from build123d import *

# Parameters (mm, degrees)
SKIZZE1_W                            = 57
SKIZZE1_H                            = 123
AUFSATZ_LINEAR_AUSTRAGEN1_DEPTH      = 2.5
SCHNITT_LINEAR_AUSTRAGEN1_DEPTH      = 84.889808678
SCHNITT_LINEAR_AUSTRAGEN2_DEPTH      = 68.828828679
SCHNITT_LINEAR_AUSTRAGEN3_DEPTH      = 70.726045338
SCHNITT_LINEAR_AUSTRAGEN3_DEPTH_BACK = 70.726045338
SCHNITT_LINEAR_AUSTRAGEN4_DEPTH      = 70.47454308
SCHNITT_LINEAR_AUSTRAGEN4_DEPTH_BACK = 70.47454308
SKIZZE9_W                            = 45.241474544
SKIZZE9_H                            = 11.280630507
AUFSATZ_LINEAR_AUSTRAGEN2_DEPTH      = 13
SCHNITT_LINEAR_AUSTRAGEN5_DEPTH      = 20
SKIZZE12_W                           = 36.023643564
SKIZZE12_H                           = 10.472363364
AUFSATZ_LINEAR_AUSTRAGEN3_DEPTH      = 5
SCHNITT_LINEAR_AUSTRAGEN6_DEPTH      = 12
SCHNITT_LINEAR_AUSTRAGEN8_DEPTH      = 0.5
SCHNITT_LINEAR_AUSTRAGEN8_DEPTH_BACK = 1.6
SKIZZE16_R                           = 3.1
SCHNITT_LINEAR_AUSTRAGEN9_DEPTH      = 1.1
SCHNITT_LINEAR_AUSTRAGEN9_DEPTH_BACK = 1
SKIZZE17_R                           = 3.1


with BuildPart() as part:
    # Skizze1 → Aufsatz-Linear austragen1 (new body)
    with BuildSketch(Plane(origin=(0, 0, 0), x_dir=(1, 0, 0), z_dir=(0, 1, 0))):
        Rectangle(SKIZZE1_W, SKIZZE1_H)
    extrude(amount=AUFSATZ_LINEAR_AUSTRAGEN1_DEPTH)

    # Skizze2 → Schnitt-Linear austragen1 (cut, through all)
    with BuildSketch(Plane(origin=(28.5, 0, 0), x_dir=(0, 0, -1), z_dir=(1, 0, 0))):
        Polygon((-61.5, 2.5), (-61.5, 0), (-60.968608596, 0), align=None)
    extrude(amount=-SCHNITT_LINEAR_AUSTRAGEN1_DEPTH, mode=Mode.SUBTRACT)

    # Skizze3 → Schnitt-Linear austragen2 (cut, through all)
    with BuildSketch(Plane(origin=(0, 2.5, 0), x_dir=(1, 0, 0), z_dir=(0, 1, 0))):
        Polygon((-28.5, -61.5), (-17.738894386, 61.5), (-28.5, 61.5), align=None)
        Polygon((28.5, -61.5), (17.738894386, 61.5), (28.5, 61.5), align=None)
    extrude(amount=-SCHNITT_LINEAR_AUSTRAGEN2_DEPTH, mode=Mode.SUBTRACT)

    # Skizze5 → Schnitt-Linear austragen3 (cut, two sides: drawn at the far end of the back side and taken through both)
    with BuildSketch(Plane(origin=(0.175618176, 0, 2.007324937), x_dir=(0, -1, 0), z_dir=(0.08715574274765484, 0, 0.9961946980917459)).offset(-SCHNITT_LINEAR_AUSTRAGEN3_DEPTH_BACK)):
        Polygon((0.008562414, 23.031470717), (-2.5, 23.031470717), (0, 21.995936811), align=None)
    extrude(amount=SCHNITT_LINEAR_AUSTRAGEN3_DEPTH + SCHNITT_LINEAR_AUSTRAGEN3_DEPTH_BACK, mode=Mode.SUBTRACT)

    # Skizze6 → Schnitt-Linear austragen4 (cut, two sides: drawn at the far end of the back side and taken through both)
    with BuildSketch(Plane(origin=(-0.152372814, 0, 1.741629235), x_dir=(0, 1, 0), z_dir=(-0.08715574274766175, 0, 0.9961946980917452)).offset(-SCHNITT_LINEAR_AUSTRAGEN4_DEPTH_BACK)):
        Polygon((2.5, 23.031470717), (0, 21.995936811), (0, 23.031470717), align=None)
    extrude(amount=SCHNITT_LINEAR_AUSTRAGEN4_DEPTH + SCHNITT_LINEAR_AUSTRAGEN4_DEPTH_BACK, mode=Mode.SUBTRACT)

    # Skizze9 → Aufsatz-Linear austragen2 (add)
    with BuildSketch(Plane.XZ):
        with Locations((0, 52.468608596)):
            Rectangle(SKIZZE9_W, SKIZZE9_H)
    extrude(amount=AUFSATZ_LINEAR_AUSTRAGEN2_DEPTH)

    # Skizze11 → Schnitt-Linear austragen5 (cut)
    with BuildSketch(Plane(origin=(0, 0, 46.828293342), x_dir=(-1, 0, 0), z_dir=(0, 0, -1))):
        Polygon((-22.620737272, -9.484039906), (0, 0), (22.620737272, -9.484039906), (22.620737272, -13), (-22.620737272, -13), align=None)
    extrude(amount=-SCHNITT_LINEAR_AUSTRAGEN5_DEPTH, mode=Mode.SUBTRACT)

    # Skizze12 → Aufsatz-Linear austragen3 (add)
    with BuildSketch(Plane.XZ):
        with Locations((0, -20.5)):
            Rectangle(SKIZZE12_W, SKIZZE12_H)
    extrude(amount=AUFSATZ_LINEAR_AUSTRAGEN3_DEPTH)

    # Skizze13 → Schnitt-Linear austragen6 (cut)
    with BuildSketch(Plane(origin=(0, 0, -25.736181682), x_dir=(-1, 0, 0), z_dir=(0, 0, -1))):
        Polygon((-18.011821782, -2.5), (-7.183132097, 0), (7.183132097, 0), (18.011821782, -2.5), (18.011821782, -5), (-18.011821782, -5), align=None)
    extrude(amount=-SCHNITT_LINEAR_AUSTRAGEN6_DEPTH, mode=Mode.SUBTRACT)

    # Skizze16 → Schnitt-Linear austragen8 (cut, two sides: drawn at the far end of the back side and taken through both)
    with BuildSketch(Plane.XZ.offset(-SCHNITT_LINEAR_AUSTRAGEN8_DEPTH_BACK)):
        with Locations(Location((12.59747694, -20.5, 0), (0, 0, 270))):
            Circle(SKIZZE16_R)
        with Locations(Location((-12.59747694, -20.5, 0), (0, 0, 270))):
            Circle(SKIZZE16_R)
    extrude(amount=SCHNITT_LINEAR_AUSTRAGEN8_DEPTH + SCHNITT_LINEAR_AUSTRAGEN8_DEPTH_BACK, mode=Mode.SUBTRACT)

    # Skizze17 → Schnitt-Linear austragen9 (cut, two sides: drawn at the far end of the back side and taken through both)
    with BuildSketch(Plane(origin=(0, -4.742019953, 0), x_dir=(1, 0, 0), z_dir=(0, 1, 0)).offset(-SCHNITT_LINEAR_AUSTRAGEN9_DEPTH_BACK)):
        with Locations(Location((-16.965552954, -52.468608596, 0), (0, 0, 270))):
            Circle(SKIZZE17_R)
        with Locations(Location((16.965552954, -52.468608596, 0), (0, 0, 270))):
            Circle(SKIZZE17_R)
    extrude(amount=SCHNITT_LINEAR_AUSTRAGEN9_DEPTH + SCHNITT_LINEAR_AUSTRAGEN9_DEPTH_BACK, mode=Mode.SUBTRACT)


solid = part.part
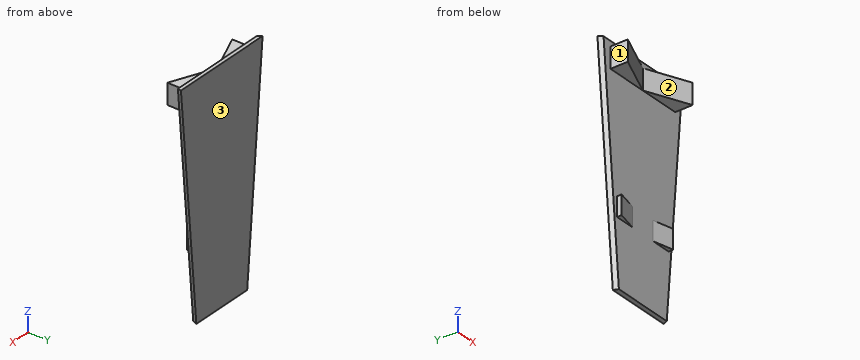
Geometry: final body of the model. Coordinates: model frame, mm. Face numbers are marked on the shaded views. Coordinates: 2 decimals unless noted, no trailing zeros. Loops run counter-clockwise (first coordinate to the right, second up) from the corner with the lowest first, then second, coordinate; pieces in that order, holes last. Notation, with made-up numbers: M 86.5,87.25 L 90.5,87.25 A28 cw 90.5,105.25 Z; hole C -3.75,44 d5. An arc over 180 degrees is marked long. One line per item, written item: value. Start each with the question number.
1) Pin query (flat end, axial travel): P1, Ø3, axis at x = -4, z = -43, coming from the -Y side; P2, Ø3, axis at x = -16, z = 53, coming from the -Y side; P3, Ø4.5, axis at x = 8.5, y = -2.5, coming from the +Z side. Return the tip coordinate at first contact, or that it passes through.
2) Cut plane C-C (z = -34.5). Return loops of the section in (x, y).
3) Cut plane B-B (x = 3). Return loops of the section in (y, z), then the cut area to 3 significant figures.
4) Material intervals for L1, parallel to X at y = 0.75, z = -20.5; L2, parallel to Z at x = 17, y = -2; L3, parallel to Z at x = -22, y = -3.5, sorted ascending. Write a range as from..to.
5) Cut plane A-A (z = -20.5). Return loops of the section in (x, y).
6) Draft query along X for the marked faces 1, 2 and 3. Return one class per face: released by +X, released by -X, zero draft, split by the parting line, or undercut.
Evaluation:
1. P1: y = 0
1. P2: y = -7.34
1. P3: z = 58.11
2. outline: M -20.1,2.5 L -19.06,0 L 19.06,0 L 20.1,2.5 Z
3. outline: M -1.26,46.83 L 0,46.83 L 0,-61.5 L 2.5,-61.5 L 2.5,61.5 L 0,60.97 L 0,58.11 L -1.26,58.11 Z
3. area: 321 mm^2
4. L1: -20.6..-15.7, -9.5..9.5, 15.7..20.6
4. L2: -25.74..-15.26, 46.83..58.11
4. L3: 46.83..58.11
5. outline: M -21.33,2.5 L -20.29,0 L -18.01,0 L -18.01,-2.5 L -7.18,0 L 7.18,0 L 18.01,-2.5 L 18.01,0 L 20.29,0 L 21.33,2.5 Z; hole M -15.7,-0.5 L -9.5,-0.5 L -9.5,1.6 L -15.7,1.6 Z; hole M 9.5,-0.5 L 15.7,-0.5 L 15.7,1.6 L 9.5,1.6 Z
6. face 1: released by -X
6. face 2: undercut
6. face 3: zero draft
